Source: CAD feature listing. Evaluate the final solid. Frame: model axes, mm. Face numbers are marked on the shaded views. Give positions to 0.01 mm unless a question says otherwise; leave off trailing zeros. Loops run counter-clockwise (first coordinate to the right, second up) from the corner with the lowest first, then second, coordinate; pieces in that order, holes last.
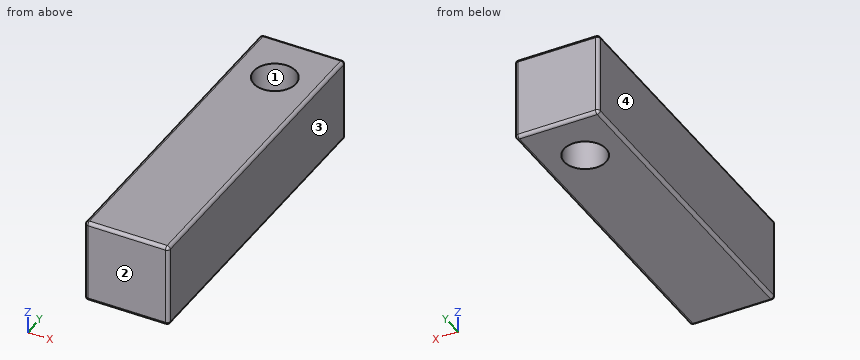
from build123d import *

# Parameters (mm, degrees)
SKIZZE1_W                       = 8
SKIZZE1_H                       = 8
AUFSATZ_LINEAR_AUSTRAGEN1_DEPTH = 31
VERRUNDUNG1_R                   = 0.3
SKIZZE2_R                       = 2
SCHNITT_LINEAR_AUSTRAGEN1_DEPTH = 9


with BuildPart() as part:
    # Skizze1 → Aufsatz-Linear austragen1 (new body)
    with BuildSketch(Plane(origin=(0, 0, 0), x_dir=(1, 0, 0), z_dir=(0, 1, 0))):
        Rectangle(SKIZZE1_W, SKIZZE1_H)
    extrude(amount=AUFSATZ_LINEAR_AUSTRAGEN1_DEPTH)

    # Verrundung1
    verrundung1_edges = [part.edges().sort_by_distance(p)[0] for p in [
        (-4, 31, 0),
        (0, 31, 4),
        (4, 31, 0),
        (0, 0, 4),
        (-4, 0, 0),
        (0, 0, -4),
        (4, 0, 0),
        (0, 31, -4),
        (4, 15.5, 4),
        (-4, 15.5, 4),
        (-4, 15.5, -4),
        (4, 15.5, -4),
    ]]
    fillet(verrundung1_edges, radius=VERRUNDUNG1_R)

    # Skizze2 → Schnitt-Linear austragen1 (cut, through all)
    with BuildSketch(Plane.XY.offset(4)):
        with Locations((0, 26)):
            Circle(SKIZZE2_R)
    extrude(amount=-SCHNITT_LINEAR_AUSTRAGEN1_DEPTH, mode=Mode.SUBTRACT)


solid = part.part
1) Cut plane A-A (x = 0). Return loops of the section in (y, z), and give its area (3 significant figures).
Checks:
outline: (0, -3.7) arc R0.3 ccw to (0.3, -4) - (24, -4) - (24, 4) - (0.3, 4) arc R0.3 ccw to (0, 3.7) - close; (28, -4) - (30.7, -4) arc R0.3 ccw to (31, -3.7) - (31, 3.7) arc R0.3 ccw to (30.7, 4) - (28, 4) - close
area: 216 mm2
2) Pull-direction query (X, two-part tool) for the marked faces 1, 2, 3 and 4; classes: released by +X, released by -X, zero draft, split by the parting line, or undercut.
Checks:
face 1: undercut
face 2: zero draft
face 3: released by +X
face 4: released by -X
3) Contact query for a flat-ended pin moving along its axis: P1, Ø3, axis at x = 0, y = 26, coming from the -Z side. Output: stop coordinate, or through.
Checks:
P1: passes through
4) Cut plane C-C (z = -2). Return loops of the section in (x, y).
Checks:
outline: (-4, 0.3) arc R0.3 ccw to (-3.7, 0) - (3.7, 0) arc R0.3 ccw to (4, 0.3) - (4, 30.7) arc R0.3 ccw to (3.7, 31) - (-3.7, 31) arc R0.3 ccw to (-4, 30.7) - close; hole circle Ø4 at (0, 26)
5) Ray query, probe 1 along Y at (x, z) = (0, -2); probe 2 along Y at (x, z) = (-1.5, 0.75). Return the intervals inside material, ascending.
Checks:
probe 1: y = 0 to 24, 28 to 31
probe 2: y = 0 to 24.68, 27.32 to 31
6) Cut plane B-B (y = 26). Return loops of the section in (x, z).
Checks:
outline: (-4, -3.7) arc R0.3 ccw to (-3.7, -4) - (-2, -4) - (-2, 4) - (-3.7, 4) arc R0.3 ccw to (-4, 3.7) - close; (2, -4) - (3.7, -4) arc R0.3 ccw to (4, -3.7) - (4, 3.7) arc R0.3 ccw to (3.7, 4) - (2, 4) - close
